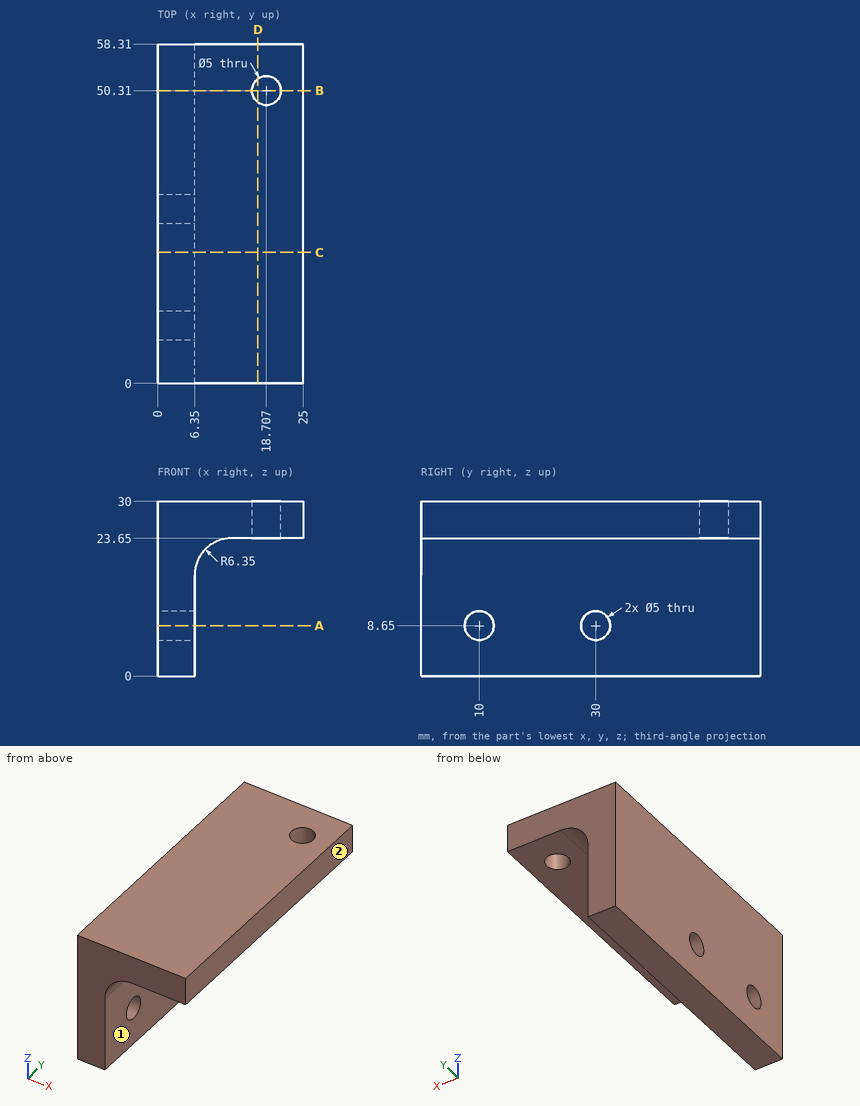
Study the drawing (mm; zero at the part's minimum x, y, z) and answer. A direction names the side the tool comes from. Round coordinates to 2 decimals unless told otherwise and drop trailing zeros. Write each loop counter-clockwise with the first axis right and the second up, starting at its lowest first coordinate (ties: lowest second). Pieces come first, ordered by that corner, then holes. Notation, with made-up numbers: (-28.75, -31.75) - (24.25, -31.75) arc R30 ccw to (24.25, -4.75) - close; hole circle Ø11 at (80, -11.75). An arc over 180 degrees is marked (long way). Use a Markdown table: item, result. Add a question column.
1. The part is cut by section C-C (y = 22.5). Write down the section's boundary in (x, z), and give its area (3 significant figures).
2. The part is cut by section A-A (z = 8.65). Write down the section's boundary in (x, y), and give its area (3 significant figures).
3. A tool of negligible diameter and unlimited length cuts with its end or side. For the marked faces 1 and 2, from which of +Z, -Z, +X, -X, +Y, -Y can it reach the whole face along a straight path? Write none if from no direction.
4. Consider line 1 (Y direction, x = 2.25, z = 8.65); line 2 (Y direction, x = 1.5, z = 10) (1 decimal); line 3 (Z direction, x = 3.75, y = 30). Determine where each line is inside the solid, lowest interval first.
5. The part is cut by section D-D (x = 17.25). Write down the section's boundary in (y, z).
6. Flat-ended cylindrical pins translate along their axes: P1, Ø8, axis at x = 18.71, y = 50.31, coming from the -Z side; P2, Ø5, axis at y = 36.5, z = 7, coming from the +X side; P3, Ø10, axis at x = 18, z = 18.5, coming from the -Y side. Find the tip coordinate at first contact, or state that the pin passes through.
7. The part is cut by section B-B (y = 50.31). Write down the section's boundary in (x, z).
Reported:
| question | item | result |
|---|---|---|
| 1 | outline | (0, 0) - (6.35, 0) - (6.35, 17.3) arc R6.35 cw to (12.7, 23.65) - (25, 23.65) - (25, 30) - (0, 30) - close |
| 1 | area | 318 mm^2 |
| 2 | outline | (0, 0) - (6.35, 0) - (6.35, 7.5) - (0, 7.5) - close; (0, 12.5) - (6.35, 12.5) - (6.35, 27.5) - (0, 27.5) - close; (0, 32.5) - (6.35, 32.5) - (6.35, 58.31) - (0, 58.31) - close |
| 2 | area | 307 mm^2 |
| 3 | face 1 | -Z, +X, +Y, -Y |
| 3 | face 2 | +Z, -Z, +X, +Y, -Y |
| 4 | line 1 | 0 to 7.5, 12.5 to 27.5, 32.5 to 58.31 |
| 4 | line 2 | 0 to 7.9, 12.1 to 27.9, 32.1 to 58.3 |
| 4 | line 3 | 0 to 6.15, 11.15 to 30 |
| 5 | outline | (0, 23.65) - (48.28, 23.65) - (48.28, 30) - (0, 30) - close; (52.34, 23.65) - (58.31, 23.65) - (58.31, 30) - (52.34, 30) - close |
| 6 | P1 | z = 23.65 |
| 6 | P2 | x = 6.35 |
| 6 | P3 | through |
| 7 | outline | (0, 0) - (6.35, 0) - (6.35, 17.3) arc R6.35 cw to (12.7, 23.65) - (16.21, 23.65) - (16.21, 30) - (0, 30) - close; (21.21, 23.65) - (25, 23.65) - (25, 30) - (21.21, 30) - close |
